from build123d import *

# Parameters (mm, degrees)
SKETCH1_W           = 31.75
SKETCH1_H           = 31.75
BOSS_EXTRUDE1_DEPTH = 3.175
SKETCH3_R           = 2.4765
CUT_EXTRUDE2_DEPTH  = 4.175
SKETCH2_R           = 3.81
CUT_EXTRUDE4_DEPTH  = 4.175
CUT_EXTRUDE5_DEPTH  = 4.175
FILLET1_R           = 6.35


with BuildPart() as part:
    # Sketch1 → Boss-Extrude1 (new body)
    with BuildSketch(Plane(origin=(0, 0, 0), x_dir=(1, 0, 0), z_dir=(0, 1, 0))):
        Rectangle(SKETCH1_W, SKETCH1_H)
    extrude(amount=BOSS_EXTRUDE1_DEPTH)

    # Sketch3 → Cut-Extrude2 (cut, through all)
    with BuildSketch(Plane.XZ):
        with Locations((-10.262339924, 10.262339924)):
            Circle(SKETCH3_R)
        with Locations((10.262339924, -10.262339924)):
            Circle(SKETCH3_R)
    extrude(amount=-CUT_EXTRUDE2_DEPTH, mode=Mode.SUBTRACT)

    # Sketch2 → Cut-Extrude4 (cut, through all)
    with BuildSketch(Plane.XZ):
        Circle(SKETCH2_R)
    extrude(amount=-CUT_EXTRUDE4_DEPTH, mode=Mode.SUBTRACT)

    # Sketch4 → Cut-Extrude5 (cut, through all)
    with BuildSketch(Plane(origin=(0, 3.175, 0), x_dir=(1, 0, 0), z_dir=(0, 1, 0))):
        Polygon((-15.875, 15.875), (-3.175, 15.875), (-15.875, 3.175), align=None)
        Polygon((15.875, -15.875), (15.875, -3.175), (3.175, -15.875), align=None)
    extrude(amount=-CUT_EXTRUDE5_DEPTH, mode=Mode.SUBTRACT)

    # Fillet1
    fillet1_edges = [part.edges().sort_by_distance(p)[0] for p in [
        (-15.875, 1.5875, -3.175),
        (-3.175, 1.5875, -15.875),
        (3.175, 1.5875, 15.875),
        (15.875, 1.5875, 3.175),
        (-15.875, 1.5875, 15.875),
        (15.875, 1.5875, -15.875),
    ]]
    fillet(fillet1_edges, radius=FILLET1_R)


solid = part.part
Geometry check sheet. Reference: the model listing, model coordinates, mm. Give positions to 0.01 mm unless a question says otherwise; leave off trailing zeros. Order: outer loops, then holes, each group sorted by start corner. A loop starts at its lowest first (then second) coordinate and runs counter-clockwise, first axis right, second up.
1) Material ranges on probe 1 along Z at (x, y) = (0, 1.35) (3 decimals); probe 2 along X at (y, z) = (0.65, 1) (3 decimals); probe 3 along Z at (x, y) = (-11.5, 1.45), recorded low to high.
Results are:
probe 1: z = -15.875 to -3.81, 3.81 to 15.875
probe 2: x = -15.875 to -3.676, 3.676 to 15.859
probe 3: z = -7.55 to 8.12, 12.41 to 15.56
2) Gauge pin test, flat ends, axial feed: pin 1 (1.5 mm diameter, centred on x = -2.5, y = 1, fed in from -Z); pin 2 (1 mm diameter, centred on y = 1.5, z = 8.5, fed in from +X). Record the tip position at first contact, or that the pin passes through.
Results are:
pin 1: stops at z = -15.76
pin 2: stops at x = 11.05
3) Cross-section at D-D (x = 5.5). Record the boundary of the cut face in (y, z) (3 decimals).
Results are:
outline: (0, -15.875) - (3.175, -15.875) - (3.175, 13.55) - (0, 13.55) - close
4) Cross-section at C-C (y = 1.5). Give the number of separate pieces and of enclosed holes in the cut face, then the cut area to 3 significant figures.
Results are:
separate pieces: 1
enclosed holes: 3
area: 742 mm2
5) Cross-section at A-A (z = 0). Record the boundary of the cut face in (x, y) (3 decimals), then the cut area to 3 significant figures.
Results are:
outline: (-15.875, 0) - (-3.81, 0) - (-3.81, 3.175) - (-15.875, 3.175) - close; (3.81, 0) - (15.875, 0) - (15.875, 3.175) - (3.81, 3.175) - close
area: 76.6 mm2
6) Cross-section at B-B (x = 0). Record the boundary of the cut face in (y, z) (3 decimals), then the cut area to 3 significant figures.
Results are:
outline: (0, -15.875) - (3.175, -15.875) - (3.175, -3.81) - (0, -3.81) - close; (0, 3.81) - (3.175, 3.81) - (3.175, 15.875) - (0, 15.875) - close
area: 76.6 mm2
7) Draft check along X on faces 1 (the cylindrical face through (-15.405, 1.565, -2.942)), 2 (the cylindrical face through (2.942, 1.565, 15.405)), 3 (the cylindrical face through (12.624, 1.565, -9.518)). Enter one of: released by +X, released by -X, zero draft, split by the parting line, or undercut.
Results are:
face 1: released by -X
face 2: released by +X
face 3: undercut
